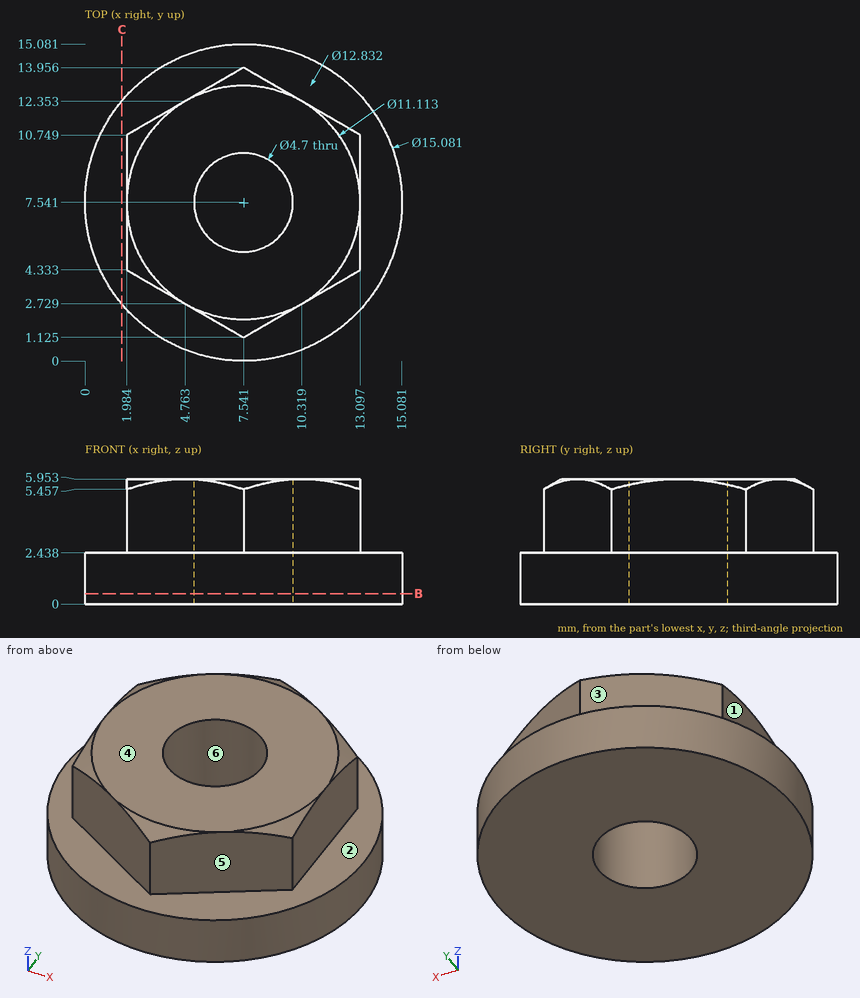
Input: dimensioned drawing with shaded views. Units: mm. Origin: part minimum x, y, z. A direction names the side the tool comes from. Coordinates: 2 decimals unless noted, no trailing zeros. Order: outer loops, then holes, each group sorted by start corner. A loop starts at its lowest first (then second) coordinate and runs counter-clockwise, first axis right, second up. Notation, with made-up numbers: (1, 67) -> (42, 67) arc R28 cw to (42, 102) -> close; hole circle Ø4 at (89, -33). An arc over 180 degrees is marked (long way). Use CSV: the item, a comma, the result in double quotes.
1) Pin query (flat end, axial travel): pin 1 Ø3 at (y, z) = (6.5, 4.5) entering from +X; pin 2 Ø1 at (x, z) = (11.5, 1) entering from +Y; pin 3 Ø1.5 at (y, z) = (12, 2) entering from -X (1 decimal). Return the tip coordinate at first contact, or that it passes through.
Findings:
pin 1,"stops at x = 13.1"
pin 2,"stops at y = 14.24"
pin 3,"stops at x = 1"
2) Section C-C on x = 1.75. Output: boundary loops of the cut face in (y, z).
Findings:
outline,"(2.71, 0) -> (12.37, 0) -> (12.37, 2.44) -> (2.71, 2.44) -> close"
3) Line query: line 1 (Y direction, x = 6, z = 3.35) (1 decimal); line 2 (Y direction, x = 11.5, z = 2.25) (1 decimal); line 3 (Z direction, x = 9.75, y = 14.5). Output: solid intervals per line, ascending.
Findings:
line 1,"y = 2 to 5.8, 9.3 to 13.1"
line 2,"y = 1.1 to 14"
line 3,"z = 0 to 2.44"
4) Section B-B on z = 0.5. Output: boundary loops of the cut face in (x, y), then the cut area to 3 significant figures.
Findings:
outline,"circle Ø15.08 at (7.54, 7.54); hole circle Ø4.7 at (7.54, 7.54)"
area,"161 mm^2"
5) Access query for the marked faces 1, 2 and 3. Directions: +Z, -Z, +X, -X, +Y, -Y. A direction counts if a zero-diameter tool reaches every point of the face in a straight line with its end or side. Return the directions, or none.
Findings:
face 1,"+Z, -X, +Y, -Y"
face 2,"+Z"
face 3,"+Z, -X, +Y"
6) Mould query, pull axis X, two halves, no side actions, for the marked faces 4, 5 and 6. Classes: +X half, -X half, draft (parallel to the pull), parting line (faces both ways), or undercut.
Findings:
face 4,"draft"
face 5,"+X half"
face 6,"undercut"
